Read the model definition and answer for the solid it produces. Units are mm, in the model's axes. Give positions to 0.01 mm unless a question says otherwise; leave off trailing zeros. Put each result on its own line as item: value. Start each with the question number.
1. A cutting plane is placed at A-A, the plane z = 197.5. Count the separate pieces of the cut face and the enclosed holes in it, plus the area to 3 significant figures.
2. Given pin 1 Ø1.9 at (x, z) = (-8, 721) entering from +Y; pin 2 Ø0.7 at (x, z) = (12, 401.5) entering from -Y; pin 3 Ø0.7 at (x, z) = (14, 286.5) entering from -Y, each flat-ended and moving along its own axis, determine where each tip first touches the part or whether it passes through.
3. For a pull along Z with two mould halves and no side action, classify faces 1 (the flat face through (5, 5, 1000)), 2 (the flat face through (5, 5, 0)) as released by +Z, released by -Z, zero draft, split by the parting line, or undercut.
4. Consider L1, parallel to X at y = -0.75, z = 332; L2, parallel to Y at x = -14.5, z = 419.5; L3, parallel to X at y = -3, z = 325. Determine where each line is inside the solid, lowest interval first. Write a range as from..to.
```python
from build123d import *

# Parameters (mm, degrees)
SKETCH1_R           = 2
BOSS_EXTRUDE1_DEPTH = 1000


with BuildPart() as part:
    # Sketch1 → Boss-Extrude1 (new body)
    with BuildSketch(Plane.XY):
        Polygon((-5.389620664, 10), (5.389620664, 10), (6.9, 8.2), (4.5, 8.2), (4.5, 6.556171609), (7.151917065, 3.899773171), (9.480384758, 3.899773171), (10, 3.599773171), (10.519615242, 3.899773171), (12.848082935, 3.899773171), (15.5, 6.556171609), (15.5, 8.2), (13.1, 8.2), (14.610379336, 10), (20, 10), (20, 4.610379336), (18.2, 3.1), (18.2, 5.5), (16.556171609, 5.5), (13.9, 2.839339828), (13.9, 0.519615231), (13.599999981, 0), (13.9, -0.519615231), (13.9, -2.839339828), (16.556171609, -5.5), (18.2, -5.5), (18.2, -3.1), (20, -4.610379336), (20, -10), (14.610379336, -10), (13.1, -8.2), (15.5, -8.2), (15.5, -6.556171609), (12.839339828, -3.9), (10.519222362, -3.9), (10, -3.600226829), (9.480777638, -3.9), (7.160660172, -3.9), (4.5, -6.556171609), (4.5, -8.2), (6.9, -8.2), (5.389620664, -10), (-5.389620664, -10), (-6.9, -8.2), (-4.5, -8.2), (-4.5, -6.556171609), (-7.160432959, -3.900226829), (-9.480384758, -3.900226829), (-10, -3.600226829), (-10.519615242, -3.900226829), (-12.839339828, -3.9), (-15.5, -6.556171609), (-15.5, -8.2), (-13.1, -8.2), (-14.610379336, -10), (-20, -10), (-20, -4.610379336), (-18.2, -3.1), (-18.2, -5.5), (-16.556171609, -5.5), (-13.9, -2.839339828), (-13.9, -0.519615231), (-13.599999981, 0), (-13.9, 0.519615231), (-13.9, 2.839339828), (-16.556171609, 5.5), (-18.2, 5.5), (-18.2, 3.1), (-20, 4.610379336), (-20, 10), (-14.610379336, 10), (-13.1, 8.2), (-15.5, 8.2), (-15.5, 6.556171609), (-12.839339828, 3.9), (-10.519615242, 3.899773171), (-10, 3.599773171), (-9.480384758, 3.899773171), (-7.160660172, 3.9), (-4.5, 6.556171609), (-4.5, 8.2), (-6.9, 8.2), align=None)
        with Locations((-10, 0)):
            Circle(SKETCH1_R, mode=Mode.SUBTRACT)
        with Locations((10, 0)):
            Circle(SKETCH1_R, mode=Mode.SUBTRACT)
        Polygon((-6.1, -2.839339828), (-2.376887287, -6.556171609), (-2.376887287, -8.2), (2.376887287, -8.2), (2.376887287, -6.556171609), (6.1, -2.839339828), (6.1, 2.839339828), (2.383168219, 6.556171609), (2.383168219, 8.2), (-2.383168219, 8.2), (-2.383168219, 6.556171609), (-6.1, 2.839339828), align=None, mode=Mode.SUBTRACT)
    extrude(amount=BOSS_EXTRUDE1_DEPTH)


solid = part.part
```
Return value:
1. separate pieces: 1
1. enclosed holes: 3
1. area: 301 mm2
2. pin 1: stops at y = 4.01
2. pin 2: stops at y = -3.9
2. pin 3: stops at y = -9.69
3. face 1: released by +Z
3. face 2: released by -Z
4. L1: x = -13.9..-11.85, -8.15..-6.1, 6.1..8.15, 11.85..13.9
4. L2: y = -9.87..-8.2, -5.56..-3.44, 3.44..5.56, 8.2..9.87
4. L3: x = -14.06..-5.94, 5.94..14.06
